Model file for the job. Use its own axes, mm. Round coordinates to 2 decimals unless told otherwise and drop trailing zeros. Order: outer loops, then holes, each group sorted by start corner. A loop starts at its lowest first (then second) coordinate and runs counter-clockwise, first axis right, second up. Notation, with made-up numbers: (70.25, 5) -> (111.25, 5) arc R28 ccw to (111.25, 32) -> close; hole circle Ø1 at (-6, 23). An arc over 180 degrees is marked (long way). Use CSV: the item, a comma, the result in double quotes.
```python
from build123d import *

# Parameters (mm, degrees)
CROQUIS1_R              = 75
SALIENTE_EXTRUIR1_DEPTH = 5
CROQUIS2_R              = 1.5
CORTAR_EXTRUIR1_DEPTH   = 107.183802908


with BuildPart() as part:
    # Croquis1 → Saliente-Extruir1 (new body)
    with BuildSketch(Plane.XY):
        Circle(CROQUIS1_R)
    extrude(amount=SALIENTE_EXTRUIR1_DEPTH)

    # Croquis2 → Cortar-Extruir1 (cut, through all)
    with BuildSketch(Plane.XY.offset(5)):
        with Locations((-50, 20)):
            Circle(CROQUIS2_R)
        with Locations(Location((-50, -20, 0), (0, 0, 180))):
            Circle(CROQUIS2_R)
        with Locations((50, -20)):
            Circle(CROQUIS2_R)
        with Locations(Location((50, 20, 0), (0, 0, 180))):
            Circle(CROQUIS2_R)
        with Locations((21, 23.876)):
            Circle(CROQUIS2_R)
        with Locations((-21, 23.876)):
            Circle(CROQUIS2_R)
        with Locations((-21, -23.8)):
            Circle(CROQUIS2_R)
        with Locations((21, -23.8)):
            Circle(CROQUIS2_R)
    extrude(amount=-CORTAR_EXTRUIR1_DEPTH, mode=Mode.SUBTRACT)


solid = part.part
```
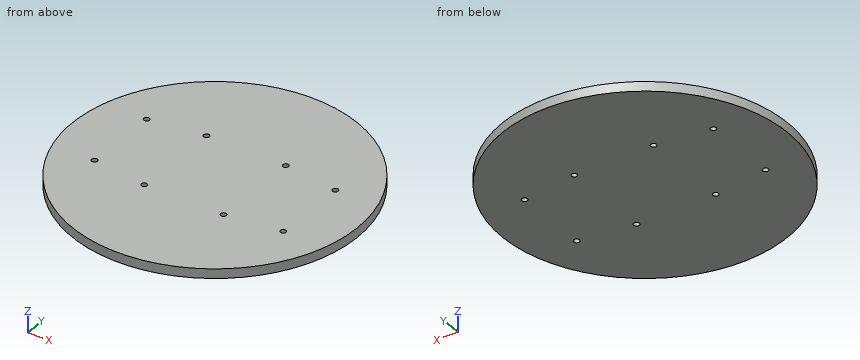
Q1. Cut at A-A (z = 2.9). State how many separate pieces and enclosed holes the cut face has, plus the area to 3 significant figures.
From the geometry:
separate pieces,"1"
enclosed holes,"8"
area,"17,600 mm²"
Q2. Cut at B-B (x = -43.5). Give the cut face in (y, z).
From the geometry:
outline,"(-61.1, 0) -> (61.1, 0) -> (61.1, 5) -> (-61.1, 5) -> close"
Q3. Cut at C-C (y = -44). Give the cut face in (x, z), plus the area to 3 significant figures.
From the geometry:
outline,"(-60.74, 0) -> (60.74, 0) -> (60.74, 5) -> (-60.74, 5) -> close"
area,"607 mm²"
Q4. Probe line 1 along Y through (x, z) = (50, 1.95); line 2 along X through (y, z) = (-19.5, 1.85); line 3 along Y through (x, z) = (-21, 1.4). List the from-to ranges inside material, lowest first.
From the geometry:
line 1,"y = -55.9 to -21.5, -18.5 to 18.5, 21.5 to 55.9"
line 2,"x = -72.42 to -51.41, -48.59 to 48.59, 51.41 to 72.42"
line 3,"y = -72 to -25.3, -22.3 to 22.38, 25.38 to 72"
Q5. Pin check, flat tips, straight feed: pin 1 (5 mm diameter, centred on x = 50, y = 20, fed in from -Z); pin 2 (1.5 mm diameter, centred on y = 13, z = 3, fed in from -X). Stop position of each tip, or through.
From the geometry:
pin 1,"stops at z = 0"
pin 2,"stops at x = -73.99"
